Read the model definition and answer for the solid it produces. Units are mm, in the model's axes. A direction names the side the tool comes from. Coordinates: 2 decimals unless noted, no trailing zeros. Loops run counter-clockwise (first coordinate to the right, second up) from the corner with the lowest first, then second, coordinate; pieces in that order, holes last. Notation, with made-up numbers: (-5, 88.5) -> (53, 88.5) arc R22 cw to (53, 108.5) -> close; hole circle Ø10 at (18, 60.5). An arc over 180 degrees is marked (long way). Answer as a JSON object with one key per item and string values. Group by question number.
1) Section D-D, the plane z = -6 is taken. Give the vertices of the cut face in (x, y).
2) Which of the six approach directions +Z, -Z, +X, -X, +Y, -Y give full straight-line access (tool end or side, diameter ignored) to faces 1 (the face through (7.55, -17.7, -8.26)), 2 (the face through (29.3, -29.2, -4.4)), 3 (the face through (15, -15, -4))?
3) A flat-ended cylindrical pin translates along its axis: P1, Ø3.5, axis at x = 10.5, y = -15, coming from the +Z side. Find the tip coordinate at first contact, or state that the pin passes through.
4) Section A-A, the plane z = -0.75 is taken. Give the vertices of the cut face in (x, y).
5) Determine the mould class of faces 4 (the face through (10.24, -13.017, -5.726)), 5 (the face through (30, -15, -4)), 6 (the face through (0.8, -29.3, -4.4)) for opening direction Y: released by +Y, released by -Y, zero draft, split by the parting line, or undercut.
6) Consider probe 1 along X at (y, z) = (-15, -0.9); probe 2 along Y at (x, z) = (25, -5); probe 3 along Y at (x, z) = (5, -2). Determine where each line is inside the solid, lowest interval first. Write a range as [from, to].
7) Section C-C, the plane y = -25 is taken. Give the vertices of the cut face in (x, z), plus the area to 3 significant figures.
8) Section B-B, the plane y = -15 is taken. Give the vertices of the cut face in (x, z).
from build123d import *

# Parameters (mm, degrees)
F0_W     = 30
F0_H     = 30
F0_R     = 1.65
F0_R_2   = 2
F1_DEPTH = 9
F2_DEPTH = 1.5
F3_DEPTH = 7
F4_DEPTH = 4
F5_R     = 4
F5_R_2   = 2
F6_DEPTH = 1.5
F7_DEPTH = 10
F8_SIZE  = 1.5


# Not quite as in the source:
# - a feature names something its author has since deleted; it is built from what else it names


with BuildPart() as f1:
    # F0 (on Top) → F1 (new body)
    with BuildSketch(Plane.XY):
        with Locations((15, -15)):
            Rectangle(F0_W, F0_H)
        with Locations((5, -25)):
            Circle(F0_R, mode=Mode.SUBTRACT)
        with Locations((25, -25)):
            Circle(F0_R_2, mode=Mode.SUBTRACT)
        with Locations((5, -5)):
            Circle(F0_R_2, mode=Mode.SUBTRACT)
        with BuildLine():
            Line((19.5, -23.75), (10.5, -23.75))
            ThreePointArc((10.5, -23.75), (1.75, -15), (10.5, -6.25))
            Line((10.5, -6.25), (19.5, -6.25))
            ThreePointArc((19.5, -6.25), (28.25, -15), (19.5, -23.75))
        make_face(mode=Mode.SUBTRACT)
        with Locations((25, -5)):
            Circle(F0_R, mode=Mode.SUBTRACT)
        with BuildLine():
            ThreePointArc((10.5, -6.25), (1.75, -15), (10.5, -23.75))
            Line((10.5, -23.75), (19.5, -23.75))
            ThreePointArc((19.5, -23.75), (28.25, -15), (19.5, -6.25))
            Line((19.5, -6.25), (10.5, -6.25))
        make_face()
        with BuildLine():
            ThreePointArc((10.5, -21.75), (3.75, -15), (10.5, -8.25))
            Line((10.5, -8.25), (19.5, -8.25))
            ThreePointArc((19.5, -8.25), (26.25, -15), (19.5, -21.75))
            Line((19.5, -21.75), (10.5, -21.75))
        make_face(mode=Mode.SUBTRACT)
        with BuildLine():
            Line((19.5, -8.25), (10.5, -8.25))
            ThreePointArc((10.5, -8.25), (3.75, -15), (10.5, -21.75))
            Line((10.5, -21.75), (19.5, -21.75))
            ThreePointArc((19.5, -21.75), (26.25, -15), (19.5, -8.25))
        make_face()
        with BuildLine():
            ThreePointArc((17.2443308628, -10.25927677), (24.75, -15), (17.2443308628, -19.74072323))
            ThreePointArc((17.2443308628, -19.74072323), (15, -20.75), (12.7556691372, -19.74072323))
            ThreePointArc((12.7556691372, -19.74072323), (5.25, -15), (12.7556691372, -10.25927677))
            ThreePointArc((12.7556691372, -10.25927677), (15, -9.25), (17.2443308628, -10.25927677))
        make_face(mode=Mode.SUBTRACT)
        with BuildLine():
            ThreePointArc((12.7556691372, -19.74072323), (15, -20.75), (17.2443308628, -19.74072323))
            ThreePointArc((17.2443308628, -19.74072323), (24.75, -15), (17.2443308628, -10.25927677))
            ThreePointArc((17.2443308628, -10.25927677), (15, -9.25), (12.7556691372, -10.25927677))
            ThreePointArc((12.7556691372, -10.25927677), (5.25, -15), (12.7556691372, -19.74072323))
        make_face()
        with Locations((10.5, -15)):
            Circle(F0_R_2, mode=Mode.SUBTRACT)
        with Locations((19.5, -15)):
            Circle(F0_R_2, mode=Mode.SUBTRACT)
        with Locations((19.5, -15)):
            Circle(F0_R_2)
        with Locations((25, -25)):
            Circle(F0_R_2)
        with Locations((25, -5)):
            Circle(F0_R)
    extrude(amount=-F1_DEPTH)

    # F0 (on Top) → F2 (cut)
    with BuildSketch(Plane.XY):
        with BuildLine():
            ThreePointArc((10.5, -6.25), (1.75, -15), (10.5, -23.75))
            Line((10.5, -23.75), (19.5, -23.75))
            ThreePointArc((19.5, -23.75), (28.25, -15), (19.5, -6.25))
            Line((19.5, -6.25), (10.5, -6.25))
        make_face()
        with BuildLine():
            ThreePointArc((10.5, -21.75), (3.75, -15), (10.5, -8.25))
            Line((10.5, -8.25), (19.5, -8.25))
            ThreePointArc((19.5, -8.25), (26.25, -15), (19.5, -21.75))
            Line((19.5, -21.75), (10.5, -21.75))
        make_face(mode=Mode.SUBTRACT)
    extrude(amount=-F2_DEPTH, mode=Mode.SUBTRACT)

    # F0 (on Top) → F3 (cut)
    with BuildSketch(Plane.XY):
        with Locations((19.5, -15)):
            Circle(F0_R_2)
    extrude(amount=-F3_DEPTH, mode=Mode.SUBTRACT)

    # F0 (on Top) → F4 (cut)
    with BuildSketch(Plane.XY):
        with BuildLine():
            ThreePointArc((12.7556691372, -19.74072323), (15, -20.75), (17.2443308628, -19.74072323))
            ThreePointArc((17.2443308628, -19.74072323), (24.75, -15), (17.2443308628, -10.25927677))
            ThreePointArc((17.2443308628, -10.25927677), (15, -9.25), (12.7556691372, -10.25927677))
            ThreePointArc((12.7556691372, -10.25927677), (5.25, -15), (12.7556691372, -19.74072323))
        make_face()
        with Locations((10.5, -15)):
            Circle(F0_R_2, mode=Mode.SUBTRACT)
        with Locations((19.5, -15)):
            Circle(F0_R_2, mode=Mode.SUBTRACT)
    extrude(amount=-F4_DEPTH, mode=Mode.SUBTRACT)

    # F5 (on face) → F6 (cut)
    with BuildSketch(Plane(origin=(0, 0, -9), x_dir=(1, 0, 0), z_dir=(0, 0, -1))):
        with Locations((10.5, 15)):
            Circle(F5_R)
        with Locations((10.5, 15)):
            Circle(F5_R_2, mode=Mode.SUBTRACT)
    extrude(amount=-F6_DEPTH, mode=Mode.SUBTRACT)

    # F0 (on Top) → F7 (cut)
    with BuildSketch(Plane.XY):
        with Locations((25, -25)):
            Circle(F0_R_2)
        with Locations((25, -5)):
            Circle(F0_R)
    extrude(amount=-F7_DEPTH, mode=Mode.SUBTRACT)

    # F8
    f8_edges = [f1.edges().sort_by_distance(p)[0] for p in [
        (30, -30, -4.5),
        (30, 0, -4.5),
        (0, -30, -4.5),
        (0, 0, -4.5),
    ]]
    chamfer(f8_edges, length=F8_SIZE)


solid = f1.part
Determined:
{
 "1": {"outline": "(0, -28.5) -> (1.5, -30) -> (28.5, -30) -> (30, -28.5) -> (30, -1.5) -> (28.5, 0) -> (1.5, 0) -> (0, -1.5) -> close; hole circle Ø4 at (5, -5); hole circle Ø3.3 at (5, -25); hole circle Ø4 at (10.5, -15); hole circle Ø4 at (19.5, -15); hole circle Ø4 at (25, -25); hole circle Ø3.3 at (25, -5)"},
 "2": {"face 1": "-Z", "face 2": "+Z, -Z, +X, -Y", "face 3": "+Z"},
 "3": {"P1": "through"},
 "4": {"outline": "(0, -28.5) -> (1.5, -30) -> (28.5, -30) -> (30, -28.5) -> (30, -1.5) -> (28.5, 0) -> (1.5, 0) -> (0, -1.5) -> close; (10.5, -21.75) -> (19.5, -21.75) arc R6.75 ccw to (19.5, -8.25) -> (10.5, -8.25) arc R6.75 ccw to start; hole circle Ø4 at (5, -5); hole circle Ø3.3 at (5, -25); hole (10.5, -23.75) -> (19.5, -23.75) arc R8.75 ccw to (19.5, -6.25) -> (10.5, -6.25) arc R8.75 ccw to start; hole (12.76, -19.74) arc R3 ccw to (17.24, -19.74) arc R5.25 ccw (long way) to (17.24, -10.26) arc R3 ccw to (12.76, -10.26) arc R5.25 ccw (long way) to start; hole circle Ø4 at (25, -25); hole circle Ø3.3 at (25, -5)"},
 "5": {"face 4": "undercut", "face 5": "zero draft", "face 6": "released by -Y"},
 "6": {"probe 1": "[0, 1.75], [3.75, 5.25], [24.75, 26.25], [28.25, 30]", "probe 2": "[-30, -27], [-23, -6.65], [-3.35, 0]", "probe 3": "[-30, -26.65], [-23.35, -7], [-3, 0]"},
 "7": {"outline": "(0, -9) -> (3.35, -9) -> (3.35, 0) -> (0, 0) -> close; (6.65, -9) -> (23, -9) -> (23, 0) -> (6.65, 0) -> close; (27, -9) -> (30, -9) -> (30, 0) -> (27, 0) -> close", "area": "204 mm²"},
 "8": {"outline": "(0, -9) -> (6.5, -9) -> (6.5, -7.5) -> (8.5, -7.5) -> (8.5, -4) -> (5.25, -4) -> (5.25, 0) -> (3.75, 0) -> (3.75, -1.5) -> (1.75, -1.5) -> (1.75, 0) -> (0, 0) -> close; (12.5, -7.5) -> (14.5, -7.5) -> (14.5, -9) -> (30, -9) -> (30, 0) -> (28.25, 0) -> (28.25, -1.5) -> (26.25, -1.5) -> (26.25, 0) -> (24.75, 0) -> (24.75, -4) -> (21.5, -4) -> (21.5, -7) -> (17.5, -7) -> (17.5, -4) -> (12.5, -4) -> close"}
}
